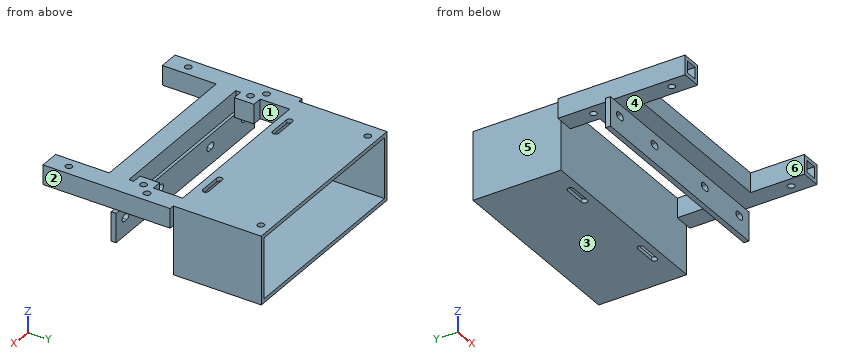
from build123d import *

# Parameters (mm, degrees)
V3_BOX_FOOTPRINT_100_X_45_MM_W                 = 100
V3_BOX_FOOTPRINT_100_X_45_MM_H                 = 45
V3_BOX_HEIGHT_35_MM_DEPTH                      = 35
V3_REAR_OPENING_96_X_31_MM_W                   = 96
V3_REAR_OPENING_96_X_31_MM_H                   = 31
V3_CAVITY_ALL_WALLS_2_MM_DEPTH                 = 43
V3_SQUARE_BEAMS_10_X_10_PITCH_95_MM_W          = 10
V3_SQUARE_BEAMS_10_X_10_PITCH_95_MM_H          = 10
V3_FORWARD_BEAM_LENGTH_65_MM_DEPTH             = 65
V3_LEFT_PCB_EAR_PROFILE_W                      = 10
V3_LEFT_PCB_EAR_PROFILE_H                      = 10
V3_LEFT_INWARD_EAR_5_MM_DEPTH                  = 5
V3_RIGHT_PCB_EAR_PROFILE_W                     = 10
V3_RIGHT_PCB_EAR_PROFILE_H                     = 10
V3_RIGHT_INWARD_EAR_5_MM_DEPTH                 = 5
V3_PCB_ROOF_PAIR_PITCH_85_MM_R                 = 1.7
V3_M3_ROOF_HOLES_DIAMETER_3_4_MM_DEPTH         = 2
V3_PCB_FORWARD_PAIR_ROW_SPACING_60_MM_R        = 1.7
V3_M3_PCB_EAR_HOLES_DEPTH                      = 10
V3_CHASSIS_TOP_HOLES_WIDTH_95_DEPTH_40_M_R     = 1.7
V3_M3_BEAM_TOP_BOTTOM_HOLES_DEPTH              = 10
V3_HANGING_PLATE_OFFSET_26_THICKNESS_2_5_W     = 110
V3_HANGING_PLATE_OFFSET_26_THICKNESS_2_5_H     = 2.5
V3_MOUNTING_PLATE_DOWNWARD_15_MM_WIDTH_1_DEPTH = 15
FOUR_HORIZONTAL_SLOTS_3_4_X_5_4_MM_DEPTH       = 2.5
CUT_EXTRUDE_1_DEPTH                            = 93.059763198
H_CROSSMEMBER_10_X_10_MM_AT_BEAM_MIDPOIN_W     = 10
H_CROSSMEMBER_10_X_10_MM_AT_BEAM_MIDPOIN_H     = 10
H_CROSSMEMBER_85_MM_DEPTH                      = 85
LONGITUDINAL_START                             = -2
BEAM_CAVITIES_6_MM_WIDE_PRESERVING_SCREW_W     = 6
BEAM_CAVITIES_6_MM_WIDE_PRESERVING_SCREW_H     = 6
BEAM_CAVITIES_6_MM_WIDE_PRESERVING_SCREW_H_2   = 27
BEAM_CAVITIES_6_MM_WIDE_PRESERVING_SCREW_H_3   = 9
LONGITUDINAL_BEAM_WALLS_2_MM_INNER_HEI_DEPTH   = 6
H_START                                        = -2
H_CROSSMEMBER_CAVITY_CONNECTS_BOTH_BEAM_W      = 89
H_CROSSMEMBER_CAVITY_CONNECTS_BOTH_BEAM_H      = 6
H_CROSSMEMBER_WALLS_2_MM_DEPTH                 = 6


with BuildPart() as part:
    # V3 box footprint 100 x 45 mm → V3 box height 35 mm (new body)
    with BuildSketch(Plane.XY):
        with Locations((0, 22.5)):
            Rectangle(V3_BOX_FOOTPRINT_100_X_45_MM_W, V3_BOX_FOOTPRINT_100_X_45_MM_H)
    extrude(amount=V3_BOX_HEIGHT_35_MM_DEPTH)

    # V3 rear opening 96 x 31 mm → V3 cavity all walls 2 mm (cut)
    with BuildSketch(Plane(origin=(0, 45, 0), x_dir=(1, 0, 0), z_dir=(0, 1, 0))):
        with Locations((0, -17.5)):
            Rectangle(V3_REAR_OPENING_96_X_31_MM_W, V3_REAR_OPENING_96_X_31_MM_H)
    extrude(amount=-V3_CAVITY_ALL_WALLS_2_MM_DEPTH, mode=Mode.SUBTRACT)

    # V3 square beams 10 x 10 pitch 95 mm → V3 forward beam length 65 mm (add)
    with BuildSketch(Plane.XZ):
        with Locations((-47.5, 30)):
            Rectangle(V3_SQUARE_BEAMS_10_X_10_PITCH_95_MM_W, V3_SQUARE_BEAMS_10_X_10_PITCH_95_MM_H)
        with Locations((47.5, 30)):
            Rectangle(V3_SQUARE_BEAMS_10_X_10_PITCH_95_MM_W, V3_SQUARE_BEAMS_10_X_10_PITCH_95_MM_H)
    extrude(amount=V3_FORWARD_BEAM_LENGTH_65_MM_DEPTH)

    # V3 left PCB ear profile → V3 left inward ear 5 mm (add)
    with BuildSketch(Plane(origin=(-42.5, 0, 0), x_dir=(0, 0, -1), z_dir=(1, 0, 0))):
        with Locations((-30, -20)):
            Rectangle(V3_LEFT_PCB_EAR_PROFILE_W, V3_LEFT_PCB_EAR_PROFILE_H)
    extrude(amount=V3_LEFT_INWARD_EAR_5_MM_DEPTH)

    # V3 right PCB ear profile → V3 right inward ear 5 mm (add)
    with BuildSketch(Plane.ZY.offset(-42.5)):
        with Locations((30, -20)):
            Rectangle(V3_RIGHT_PCB_EAR_PROFILE_W, V3_RIGHT_PCB_EAR_PROFILE_H)
    extrude(amount=V3_RIGHT_INWARD_EAR_5_MM_DEPTH)

    # V3 PCB roof pair pitch 85 mm → V3 M3 roof holes diameter 3.4 mm (cut)
    with BuildSketch(Plane.XY.offset(35)):
        with Locations((-42.5, 40)):
            Circle(V3_PCB_ROOF_PAIR_PITCH_85_MM_R)
        with Locations((42.5, 40)):
            Circle(V3_PCB_ROOF_PAIR_PITCH_85_MM_R)
    extrude(amount=-V3_M3_ROOF_HOLES_DIAMETER_3_4_MM_DEPTH, mode=Mode.SUBTRACT)

    # V3 PCB forward pair row spacing 60 mm → V3 M3 PCB ear holes (cut)
    with BuildSketch(Plane.XY.offset(35)):
        with Locations((-42.5, -20)):
            Circle(V3_PCB_FORWARD_PAIR_ROW_SPACING_60_MM_R)
        with Locations((42.5, -20)):
            Circle(V3_PCB_FORWARD_PAIR_ROW_SPACING_60_MM_R)
    extrude(amount=-V3_M3_PCB_EAR_HOLES_DEPTH, mode=Mode.SUBTRACT)

    # V3 chassis top holes width 95 depth 40 mm → V3 M3 beam top bottom holes (cut)
    with BuildSketch(Plane.XY.offset(35)):
        with Locations((-47.5, -55)):
            Circle(V3_CHASSIS_TOP_HOLES_WIDTH_95_DEPTH_40_M_R)
        with Locations((-47.5, -15)):
            Circle(V3_CHASSIS_TOP_HOLES_WIDTH_95_DEPTH_40_M_R)
        with Locations((47.5, -55)):
            Circle(V3_CHASSIS_TOP_HOLES_WIDTH_95_DEPTH_40_M_R)
        with Locations((47.5, -15)):
            Circle(V3_CHASSIS_TOP_HOLES_WIDTH_95_DEPTH_40_M_R)
    extrude(amount=-V3_M3_BEAM_TOP_BOTTOM_HOLES_DEPTH, mode=Mode.SUBTRACT)

    # V3 hanging plate offset 26 thickness 2.5 mm → V3 mounting plate downward 15 mm width 110 (add)
    with BuildSketch(Plane(origin=(0, 0, 25), x_dir=(-1, 0, 0), z_dir=(0, 0, -1))):
        with Locations((0, -27.25)):
            Rectangle(V3_HANGING_PLATE_OFFSET_26_THICKNESS_2_5_W, V3_HANGING_PLATE_OFFSET_26_THICKNESS_2_5_H)
    extrude(amount=V3_MOUNTING_PLATE_DOWNWARD_15_MM_WIDTH_1_DEPTH)

    # V3 slots 6 mm below beam underside centers 20 and 47.5 → Four horizontal slots 3.4 x 5.4 mm (cut)
    with BuildSketch(Plane.XZ.offset(28.5)):
        with BuildLine():
            Line((-48.5, 20.7), (-46.5, 20.7))
            ThreePointArc((-46.5, 20.7), (-44.8, 19), (-46.5, 17.3))
            Line((-46.5, 17.3), (-48.5, 17.3))
            ThreePointArc((-48.5, 17.3), (-50.2, 19), (-48.5, 20.7))
        make_face()
        with BuildLine():
            Line((-21, 20.7), (-19, 20.7))
            ThreePointArc((-19, 20.7), (-17.3, 19), (-19, 17.3))
            Line((-19, 17.3), (-21, 17.3))
            ThreePointArc((-21, 17.3), (-22.7, 19), (-21, 20.7))
        make_face()
        with BuildLine():
            Line((19, 20.7), (21, 20.7))
            ThreePointArc((21, 20.7), (22.7, 19), (21, 17.3))
            Line((21, 17.3), (19, 17.3))
            ThreePointArc((19, 17.3), (17.3, 19), (19, 20.7))
        make_face()
        with BuildLine():
            Line((46.5, 20.7), (48.5, 20.7))
            ThreePointArc((48.5, 20.7), (50.2, 19), (48.5, 17.3))
            Line((48.5, 17.3), (46.5, 17.3))
            ThreePointArc((46.5, 17.3), (44.8, 19), (46.5, 20.7))
        make_face()
    extrude(amount=-FOUR_HORIZONTAL_SLOTS_3_4_X_5_4_MM_DEPTH, mode=Mode.SUBTRACT)

    # 草图2 → 切除-拉伸1 (cut, through all)
    with BuildSketch(Plane(origin=(0, 0, 0), x_dir=(-1, 0, 0), z_dir=(0, 0, -1))):
        with BuildLine():
            Line((-32.029979042, 6.459471041), (-21.029979042, 6.459471041))
            ThreePointArc((-21.029979042, 6.459471041), (-19.570508001, 5), (-21.029979042, 3.540528959))
            Line((-21.029979042, 3.540528959), (-32.029979042, 3.540528959))
            ThreePointArc((-32.029979042, 3.540528959), (-33.489450083, 5), (-32.029979042, 6.459471041))
        make_face()
        with BuildLine():
            Line((23.620107008, 6.558669056), (34.620107008, 6.558669056))
            ThreePointArc((34.620107008, 6.558669056), (36.178776063, 5), (34.620107008, 3.441330944))
            Line((34.620107008, 3.441330944), (23.620107008, 3.441330944))
            ThreePointArc((23.620107008, 3.441330944), (22.061437952, 5), (23.620107008, 6.558669056))
        make_face()
    extrude(amount=-CUT_EXTRUDE_1_DEPTH, mode=Mode.SUBTRACT)

    # H crossmember 10 x 10 mm at beam midpoint → H crossmember 85 mm (add)
    with BuildSketch(Plane(origin=(-42.5, 0, 0), x_dir=(0, 0, -1), z_dir=(1, 0, 0))):
        with Locations((-30, -32.5)):
            Rectangle(H_CROSSMEMBER_10_X_10_MM_AT_BEAM_MIDPOIN_W, H_CROSSMEMBER_10_X_10_MM_AT_BEAM_MIDPOIN_H)
    extrude(amount=H_CROSSMEMBER_85_MM_DEPTH)

    # Beam cavities 6 mm wide preserving screw collars → Longitudinal beam walls 2 mm - inner height 6 mm (cut)
    with BuildSketch(Plane.XY.offset(35).offset(LONGITUDINAL_START)):
        with Locations((-47.5, -62)):
            Rectangle(BEAM_CAVITIES_6_MM_WIDE_PRESERVING_SCREW_W, BEAM_CAVITIES_6_MM_WIDE_PRESERVING_SCREW_H)
        with Locations((-47.5, -37.5)):
            Rectangle(BEAM_CAVITIES_6_MM_WIDE_PRESERVING_SCREW_W, BEAM_CAVITIES_6_MM_WIDE_PRESERVING_SCREW_H_2)
        with Locations((-47.5, -6.5)):
            Rectangle(BEAM_CAVITIES_6_MM_WIDE_PRESERVING_SCREW_W, BEAM_CAVITIES_6_MM_WIDE_PRESERVING_SCREW_H_3)
        with Locations((47.5, -62)):
            Rectangle(BEAM_CAVITIES_6_MM_WIDE_PRESERVING_SCREW_W, BEAM_CAVITIES_6_MM_WIDE_PRESERVING_SCREW_H)
        with Locations((47.5, -37.5)):
            Rectangle(BEAM_CAVITIES_6_MM_WIDE_PRESERVING_SCREW_W, BEAM_CAVITIES_6_MM_WIDE_PRESERVING_SCREW_H_2)
        with Locations((47.5, -6.5)):
            Rectangle(BEAM_CAVITIES_6_MM_WIDE_PRESERVING_SCREW_W, BEAM_CAVITIES_6_MM_WIDE_PRESERVING_SCREW_H_3)
    extrude(amount=-LONGITUDINAL_BEAM_WALLS_2_MM_INNER_HEI_DEPTH, mode=Mode.SUBTRACT)

    # H crossmember cavity connects both beam cavities → H crossmember walls 2 mm (cut)
    with BuildSketch(Plane.XY.offset(35).offset(H_START)):
        with Locations((0, -32.5)):
            Rectangle(H_CROSSMEMBER_CAVITY_CONNECTS_BOTH_BEAM_W, H_CROSSMEMBER_CAVITY_CONNECTS_BOTH_BEAM_H)
    extrude(amount=-H_CROSSMEMBER_WALLS_2_MM_DEPTH, mode=Mode.SUBTRACT)


solid = part.part
Work out the finished part from the listing and answer in its coordinate system (mm). Face numbers are marked on the shaded views. A direction names the side the tool comes from. Round coordinates to 2 decimals unless told otherwise and drop trailing zeros. Loops run counter-clockwise (first coordinate to the right, second up) from the corner with the lowest first, then second, coordinate; pieces in that order, holes last. Notation, with made-up numbers: (31, 39.5) -> (65, 39.5) arc R13 cw to (65, 44.5) -> close; hole circle Ø3 at (9, 33). An arc over 180 degrees is marked (long way). Use one line per item in the form item = value.
(1) Find section D-D on y = 5. Give the vertices of the cut face in (x, z).
Answer list:
outline = (-50, 0) -> (-36.18, 0) -> (-36.18, 2) -> (-48, 2) -> (-48, 33) -> (-36.18, 33) -> (-36.18, 35) -> (-50, 35) -> close; (-22.06, 0) -> (19.57, 0) -> (19.57, 2) -> (-22.06, 2) -> close; (-22.06, 33) -> (19.57, 33) -> (19.57, 35) -> (-22.06, 35) -> close; (33.49, 0) -> (50, 0) -> (50, 35) -> (33.49, 35) -> (33.49, 33) -> (48, 33) -> (48, 2) -> (33.49, 2) -> close
(2) Find section A-A on y = -9. Give the vertices of the cut face in (x, z), then the cut area to 3 significant figures.
Answer list:
outline = (-52.5, 25) -> (-42.5, 25) -> (-42.5, 35) -> (-52.5, 35) -> close; (42.5, 25) -> (52.5, 25) -> (52.5, 35) -> (42.5, 35) -> close; hole (-50.5, 27) -> (-44.5, 27) -> (-44.5, 33) -> (-50.5, 33) -> close; hole (44.5, 27) -> (50.5, 27) -> (50.5, 33) -> (44.5, 33) -> close
area = 128 mm2
(3) For a pull along X with two mould halves and no side action, classify the marked faces 1, 2 and 3 as released by +X, released by -X, zero draft, split by the parting line, or undercut.
Answer list:
face_1 = undercut
face_2 = released by +X
face_3 = zero draft
(4) Find section C-C on y = 40. Give the vertices of the cut face in (x, z), then the cut area to 3 significant figures.
Answer list:
outline = (-50, 0) -> (50, 0) -> (50, 35) -> (44.2, 35) -> (44.2, 33) -> (48, 33) -> (48, 2) -> (-48, 2) -> (-48, 33) -> (-44.2, 33) -> (-44.2, 35) -> (-50, 35) -> close; (-40.8, 33) -> (40.8, 33) -> (40.8, 35) -> (-40.8, 35) -> close
area = 510 mm2
(5) Straight lines are drawn through the part: line 1 (Y direction, x = -15, z = 32); line 2 (Y direction, x = 45, z = 29.5); line 3 (Y direction, x = 47.5, z = 28.75). For each, find the intervals that lie inside material, in ascending order.
Answer list:
line_1 = -37.5 to -35.5, -29.5 to -27.5, 0 to 2
line_2 = -59 to -51, -24 to -11, -2 to 2
line_3 = -59 to -56.7, -53.3 to -51, -24 to -16.7, -13.3 to -11, -2 to 2
(6) A tool of negligible diameter and unlimited length cuts with its end or side. For the marked faces 4, 5 and 6, from which of +Z, -Z, +X, -X, +Y, -Y can it reach the whole face along a straight path? Write none if from no direction.
Answer list:
face_4 = -Z, +X, -X, -Y
face_5 = +Z, -Z, -X, +Y
face_6 = +Z, -Z, -Y
(7) Flat-ended cylindrical pins translate along their axes: P1, Ø6.5, axis at x = -46, y = -62, coming from the -Z side; P2, Ø3, axis at y = -62.5, z = 29.5, coming from the +X side; P3, Ø1, axis at x = 20, y = -26.5, coming from the -Z side. Find the tip coordinate at first contact, or state that the pin passes through.
Answer list:
P1 = 25
P2 = 52.5
P3 = 10
(8) Find section B-B on x = -9. Give the vertices of the cut face in (y, z), then the cut area to 4 significant figures.
Answer list:
outline = (-37.5, 25) -> (-28.5, 25) -> (-28.5, 10) -> (-26, 10) -> (-26, 25) -> (-27.5, 25) -> (-27.5, 35) -> (-37.5, 35) -> close; (0, 0) -> (45, 0) -> (45, 2) -> (2, 2) -> (2, 33) -> (45, 33) -> (45, 35) -> (0, 35) -> close; hole (-35.5, 27) -> (-29.5, 27) -> (-29.5, 33) -> (-35.5, 33) -> close
area = 343.5 mm2
